Work out the finished part from the listing and answer in its coordinate system (mm). Face numbers are marked on the shaded views. A direction names the side the tool comes from. Round coordinates to 2 decimals unless told otherwise and drop trailing zeros. Loops run counter-clockwise (first coordinate to the right, second up) from the corner with the lowest first, then second, coordinate; pieces in that order, holes last. Notation, with made-up numbers: (-9.5, 43.5) - (7.5, 43.5) arc R4 ccw to (7.5, 48.5) - close; hole circle Ø2 at (-13.5, 44). An arc over 180 degrees is marked (long way). Return JSON: item names as keys, results as strings.
Autodesk Inventor part; units mm, degrees
ref_plane "YZ Plane" through (0, 0, 0) normal (1, 0, 0) x (0, 1, 0)
ref_plane "XZ Plane" through (0, 0, 0) normal (0, 1, 0) x (-1, 0, 0)
ref_plane "XY Plane" through (0, 0, 0) normal (0, 0, 1) x (1, 0, 0)
sketch "Sketch1" plane through (0, 0, 0) normal (1, 0, 0) x (0, 1, 0)
  line L0 (0, 0) -> (69.85, 0)
  line L1 (69.85, 0) -> (69.85, -19.05)
  line L2 (69.85, -19.05) -> (0, -19.05)
  line L3 (0, -19.05) -> (0, 0)
  dimension "d0" = 19.05
  dimension "d1" = 69.85
extrude "Extrusion1" add sketch "Sketch1" along normal blind 9.525
sketch "Sketch2" plane through (9.525, 0, 0) normal (1, 0, 0) x (0, 0, -1)
  line L0 (0, 69.85) -> (0, 0)
  line L1 (0, 0) -> (19.05, 0)
  line L2 (19.05, 0) -> (19.05, 69.85)
  line L3 (19.05, 69.85) -> (0, 69.85)
  point P0 (9.525, 66.675)
  point P1 (9.525, 39.7256)
  dimension "d4" = 26.9494
  dimension "d5" = 19.05
  dimension "d6" = 69.85
  dimension "d7" = 3.175
  dimension "d8" = 9.525
  dimension "d9" = 9.525
hole "Hole1" at (9.525, 66.675, -9.525) at (9.525, 39.7256, -9.525) direction (-1, 0, 0) diameter 3.556 depth 25.4 tip angle 118
sketch "Sketch5" plane through (0, 0, 0) normal (-1, 0, 0) x (0, 0, 1)
  circle A0 centre (-9.525, 66.675) radius 1.778
  circle A1 centre (-9.525, 39.7256) radius 1.778
  line L0 (0, 0) -> (0, 69.85)
  line L1 (0, 69.85) -> (-19.05, 69.85)
  line L2 (-19.05, 69.85) -> (-19.05, 0)
  line L3 (-19.05, 0) -> (0, 0)
  line L4 (-19.05, 0) -> (-19.05, 69.85)
  line L5 (0, 69.85) -> (0, 0)
  line L6 (-19.05, 0) -> (0, 0)
  line L7 (0, 0) -> (0, 6.35)
  line L8 (0, 6.35) -> (-19.05, 6.35)
  line L9 (-19.05, 6.35) -> (-19.05, 0)
  dimension "d31" = 6.35
extrude "Extrusion2" add sketch "Sketch5" along normal blind 12.7 contours L3 L2 L8 L0
sketch "Sketch6" plane through (0, 6.35, 0) normal (0, 1, 0) x (1, 0, 0)
  line L0 (0, 19.05) -> (0, 0)
  line L1 (0, 19.05) -> (-12.7, 19.05)
  line L2 (-12.7, 0) -> (-12.7, 19.05)
  line L3 (0, 0) -> (-12.7, 0)
  point P0 (0, 0)
  point P1 (-6.35, 13.97)
  point P2 (-6.35, 5.08)
  dimension "d34" = 19.05
  dimension "d35" = 5.08
  dimension "d36" = 5.08
hole "Hole3" at (-6.35, 6.35, -13.97) at (-6.35, 6.35, -5.08) direction (0, -1, 0) diameter 3.556 depth 25.4 tip angle 118
fillet "Fillet1" radius 3.175 1 edges at (0, 6.35, -9.525)
properties part number "GlyphtMotorBrace"
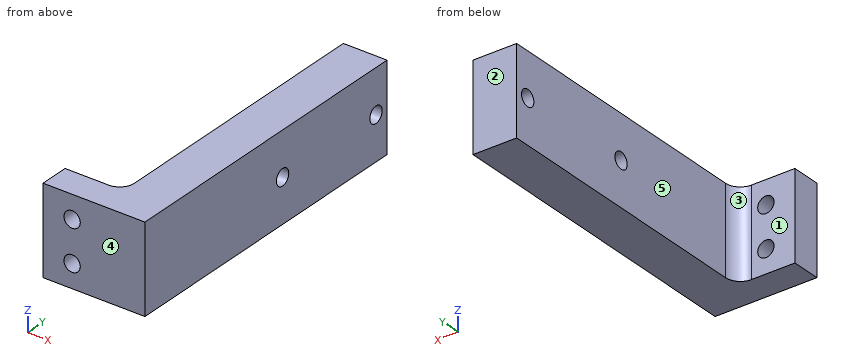
1) Flat-ended cylindrical pins translate along their axes: pin 1 (1.5 mm diameter, centred on y = 15, z = -8, fed in from -X); pin 2 (6 mm diameter, centred on x = -7.5, z = -4.5, fed in from +Y). Find the tip coordinate at first contact, or state that the pin passes through.
Verdict:
{"pin 1": "stops at x = 0", "pin 2": "stops at y = 6.35"}
2) Determine the mould class of the marked faces 3, 4 and 5 for opening direction Y: pulls with the +Y half, pulls with the -Y half, needs draft (parallel to the pull), parting line crosses it, or undercut.
Verdict:
{"face 3": "pulls with the +Y half", "face 4": "pulls with the -Y half", "face 5": "needs draft"}
3) A tool of negligible diameter and unlimited length cuts with its end or side. For the marked faces 1 and 2, from which of +Z, -Z, +X, -X, +Y, -Y can it reach the whole face along a straight path? Write none if from no direction.
Verdict:
{"face 1": "+Z, -Z, -X, +Y", "face 2": "+Z, -Z, +X, -X, +Y"}
4) Find the intervals of material crossed by L1, parallel to Z at x = -6.35, y = 5; L2, parallel to Y at x = 0.75, z = -9.5; L3, parallel to X at y = 4.25, z = -13.97 (3 decimals), in increasing order.
Verdict:
{"L1": "z = -19.05 to -15.75, -12.19 to -6.86, -3.3 to 0", "L2": "y = 0 to 37.95, 41.5 to 64.9, 68.45 to 69.85", "L3": "x = -12.7 to -8.128, -4.572 to 9.525"}
5) Section A-A (x = -6.35) is taken. Give the vertices of the cut face in (y, z).
Verdict:
{"outline": "(0, -19.05) - (6.35, -19.05) - (6.35, -15.75) - (0, -15.75) - close; (0, -12.19) - (6.35, -12.19) - (6.35, -6.86) - (0, -6.86) - close; (0, -3.3) - (6.35, -3.3) - (6.35, 0) - (0, 0) - close"}
6) Section B-B (z = -13.97) is taken. Give the vertices of the cut face in (x, y) (3 decimals).
Verdict:
{"outline": "(-12.7, 0) - (-8.128, 0) - (-8.128, 6.35) - (-12.7, 6.35) - close; (-4.572, 0) - (9.525, 0) - (9.525, 69.85) - (0, 69.85) - (0, 9.525) arc R3.175 cw to (-3.175, 6.35) - (-4.572, 6.35) - close"}
7) Section C-C (y = 44) is taken. Give the vertices of the cut face in (x, z) (3 decimals), and give its area (3 significant figures).
Verdict:
{"outline": "(0, -19.05) - (9.525, -19.05) - (9.525, 0) - (0, 0) - close", "area": "181 mm2"}
